Here's how the part is built. I have some questions about the finished solid (model axes, mm). Round coordinates to 2 decimals unless told otherwise and drop trailing zeros. Order: outer loops, then holes, each group sorted by start corner. A loop starts at its lowest first (then second) coordinate and runs counter-clockwise, first axis right, second up. Notation, with made-up numbers: (31, -16.75) -> (55, -16.75) arc R28 ccw to (55, 3.25) -> close; hole circle Ø1 at (65.5, 33). An arc over 180 degrees is marked (long way). Use a Markdown table: item, result. Add a question column.
(1) If I drill on probe 1 along Y at (x, z) = (37.5, 1); probe 2 along X at (y, z) = (-8, 1.5); probe 3 along Y at (x, z) = (11, 6), over which ranges is the centre line in solid material (lowest first)?
(2) I want a section at B-B, the plane y = -12. Please give me the cut outline in (x, z).
(3) I want a section at C-C, the plane x = 35. Please give me the cut outline in (y, z).
(4) I want a section at A-A, the plane z = 7.5. Please give me the cut outline in (x, y), then the cut area to 3 significant figures.
(5) I'm going to push a flat-ended pin straight in: P1, Ø4, axis at x = 43, z = 7, coming from the +Y side. Where does the tip first touch, or does it pass through?
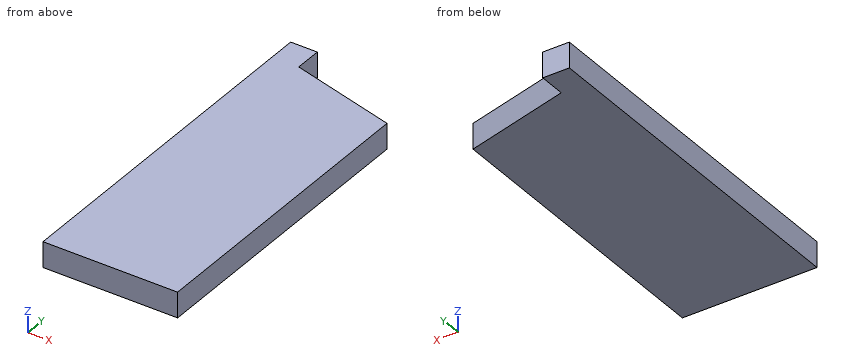
from build123d import *

# Parameters (mm, degrees)
EXTRUDE_1_DEPTH          = 9.4
CUT_EXTRUDE_1_DEPTH      = 1
CUT_EXTRUDE_1_DEPTH_BACK = 10.4


with BuildPart() as part:
    # 草图1 → 凸台-拉伸1 (new body)
    with BuildSketch(Plane.XY):
        Polygon((9.8, 0), (0, 0), (0, -133.83), (49.6, -133.83), (49.6, 0), (39.8, 0), (39.8, -10), (9.8, -10), align=None)
    extrude(amount=EXTRUDE_1_DEPTH)

    # 草图2 → 切除-拉伸1 (cut, two sides)
    with BuildSketch(Plane.XY.offset(9.4)) as cut_extrude_1_sk:
        Polygon((39.8, -10), (9.8, -10), (49.6, -20.664377859), (49.6, 0), (39.8, 0), align=None)
    extrude(amount=CUT_EXTRUDE_1_DEPTH, mode=Mode.SUBTRACT)
    extrude(cut_extrude_1_sk.sketch, amount=-CUT_EXTRUDE_1_DEPTH_BACK, mode=Mode.SUBTRACT)


solid = part.part
Taken from the geometry:
| question | item | result |
|---|---|---|
| 1 | probe 1 | y = -133.83 to -17.42 |
| 1 | probe 2 | x = 0 to 9.8 |
| 1 | probe 3 | y = -133.83 to -10.32 |
| 2 | outline | (0, 0) -> (17.26, 0) -> (17.26, 9.4) -> (0, 9.4) -> close |
| 3 | outline | (-133.83, 0) -> (-16.75, 0) -> (-16.75, 9.4) -> (-133.83, 9.4) -> close |
| 4 | outline | (0, -133.83) -> (49.6, -133.83) -> (49.6, -20.66) -> (9.8, -10) -> (9.8, 0) -> (0, 0) -> close |
| 4 | area | 6,030 mm2 |
| 5 | P1 | stops at y = -18.36 |
